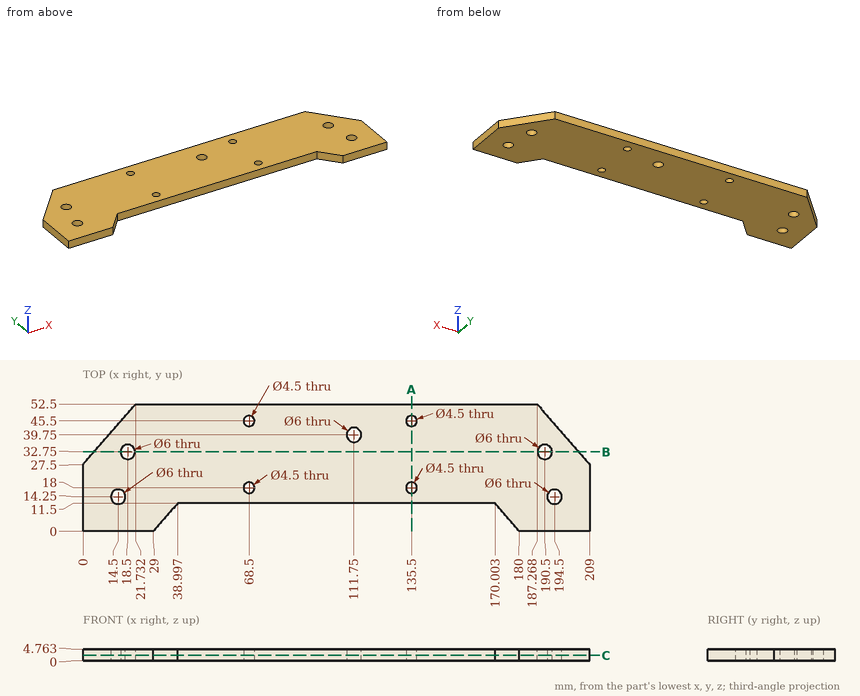
Geometry check sheet. Reference: drawing and pictorial views, mm from the part's lowest x, y, z. Give positions to 0.01 mm unless a question says otherwise; leave off trailing zeros. Order: outer loops, then holes, each group sorted by start corner. A loop starts at its lowest first (then second) coordinate and runs counter-clockwise, first axis right, second up. Notation, with made-up numbers: (9, -19) - (50, -19) arc R22 ccw to (50, 6) - close; hole circle Ø10 at (84.25, 88.5). An arc over 180 degrees is marked (long way). Answer as CSV lines item,"result".
1. Section check C-C (z = 2.3). State how many separate pieces and enclosed holes the cut face has, then the cut area to 3 significant figures.
Result sheet:
separate pieces,"1"
enclosed holes,"9"
area,"8,600 mm²"
2. Section check B-B (y = 32.75). Record the boundary of the cut face in (x, z).
Result sheet:
outline,"(4.56, 0) - (15.5, 0) - (15.5, 4.76) - (4.56, 4.76) - close; (21.5, 0) - (187.5, 0) - (187.5, 4.76) - (21.5, 4.76) - close; (193.5, 0) - (204.44, 0) - (204.44, 4.76) - (193.5, 4.76) - close"
3. Go/stop test with a flat-tipped pin: P1, Ø1.4, axis at x = 130.5, z = 3.5, coming from the -Y side. Record where the tip stops, or that it passes through.
Result sheet:
P1,"y = 11.5"
4. Section check A-A (x = 135.5). Record the boundary of the cut face in (y, z).
Result sheet:
outline,"(11.5, 0) - (15.75, 0) - (15.75, 4.76) - (11.5, 4.76) - close; (20.25, 0) - (43.25, 0) - (43.25, 4.76) - (20.25, 4.76) - close; (47.75, 0) - (52.5, 0) - (52.5, 4.76) - (47.75, 4.76) - close"
5. Scan lines: probe 1 along Y at (x, z) = (68.5, 3.4); probe 2 along Y at (x, z) = (70.5, 3.5); probe 3 along Y at (x, z) = (117.5, 3). Record each from-to range of solid material in increasing order. Write a range as from..to.
Result sheet:
probe 1,"11.5..15.75, 20.25..43.25, 47.75..52.5"
probe 2,"11.5..16.97, 19.03..44.47, 46.53..52.5"
probe 3,"11.5..52.5"
